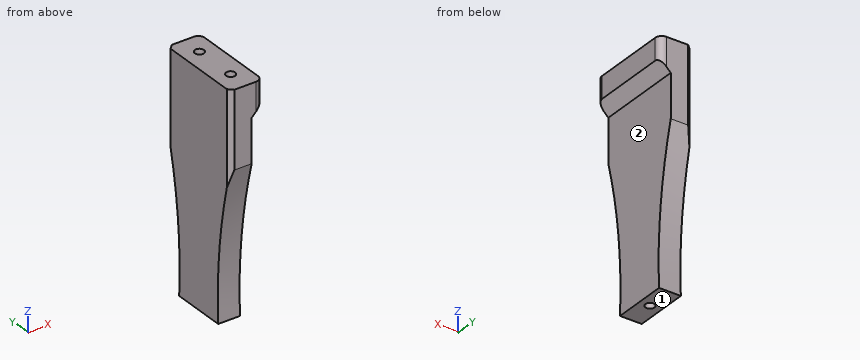
```python
from build123d import *

# Parameters (mm, degrees)
BOSS_EXTRUDE1_DEPTH   = 20
CUT_EXTRUDE1_DEPTH    = 108.935165725
FILLET2_R             = 3
M5_TAPPED_HOLE1_D     = 4.2
M5_TAPPED_HOLE1_DEPTH = 13.7381927
M5_TAPPED_HOLE1_TIP   = 1.2618073
M5_TAPPED_HOLE2_D     = 4.2
M5_TAPPED_HOLE2_DEPTH = 13.7381927
M5_TAPPED_HOLE2_TIP   = 1.2618073
CHAMFER1_SIZE         = 5
CHAMFER2_SIZE         = 2


with BuildPart() as part:
    # Sketch1 → Boss-Extrude1 (new, symmetric)
    with BuildSketch(Plane(origin=(0, 0, 0), x_dir=(1, 0, 0), z_dir=(0, 1, 0))):
        Polygon((0, 0), (15, 0), (15, 10), (10, 10), (10, 105), (0, 105), align=None)
    extrude(amount=BOSS_EXTRUDE1_DEPTH, both=True)

    # Sketch3 → Cut-Extrude1 (cut, through all)
    with BuildSketch(Plane.ZY):
        with BuildLine():
            Line((-35, -20), (-105, -20))
            Line((-105, -20), (-105, -12.5))
            add(Edge.make_bspline(
                [(-105, -12.5), (-69.476387912, -10.752287941), (-35, -20)],
                knots=[0, 0, 0, 1, 1, 1], degree=2))
        make_face()
    cut_extrude1 = extrude(amount=-CUT_EXTRUDE1_DEPTH, mode=Mode.SUBTRACT)

    # Mirror1: Cut-Extrude1 across plane
    add(cut_extrude1.mirror(Plane.ZX), mode=Mode.SUBTRACT)

    # Fillet2
    fillet2_edges = [part.edges().sort_by_distance(p)[0] for p in [
        (15, 20, -5),
        (15, -20, -5),
    ]]
    fillet(fillet2_edges, radius=FILLET2_R)

    # M5 Tapped Hole1
    with Locations(Plane(origin=(0, 0, -105), x_dir=(-1, 0, 0), z_dir=(0, 0, -1))):
        with Locations((-5.195, 0)):
            Hole(M5_TAPPED_HOLE1_D / 2, depth=M5_TAPPED_HOLE1_DEPTH)
            with Locations((0, 0, -(M5_TAPPED_HOLE1_DEPTH + M5_TAPPED_HOLE1_TIP / 2))):  # 118° drill point
                Cone(0, M5_TAPPED_HOLE1_D / 2, M5_TAPPED_HOLE1_TIP, mode=Mode.SUBTRACT)

    # M5 Tapped Hole2
    with Locations(Plane.XY):
        with Locations((7.5, -10), (7.5, 10)):
            Hole(M5_TAPPED_HOLE2_D / 2, depth=M5_TAPPED_HOLE2_DEPTH)
            with Locations((0, 0, -(M5_TAPPED_HOLE2_DEPTH + M5_TAPPED_HOLE2_TIP / 2))):  # 118° drill point
                Cone(0, M5_TAPPED_HOLE2_D / 2, M5_TAPPED_HOLE2_TIP, mode=Mode.SUBTRACT)

    # Chamfer1
    chamfer1_edges = [part.edges().sort_by_distance(p)[0] for p in [
        (10, 0, -10),
    ]]
    chamfer(chamfer1_edges, length=CHAMFER1_SIZE - 0.0001)  # a hair under: the kernel refuses the full size

    # Chamfer2
    chamfer2_edges = [part.edges().sort_by_distance(p)[0] for p in [
        (0, -20, -17.5),
        (0, 20, -17.5),
    ]]
    chamfer(chamfer2_edges, length=CHAMFER2_SIZE)


solid = part.part
```
Geometry: final body of the model. Coordinates: model frame, mm. Face numbers are marked on the shaded views. A direction names the side the tool comes from. Coordinates: 2 decimals unless noted, no trailing zeros. Loops run counter-clockwise (first coordinate to the right, second up) from the corner with the lowest first, then second, coordinate; pieces in that order, holes last. Notation, with made-up numbers: (7.25, 23.5) -> (62.25, 23.5) arc R3 ccw to (62.25, 27.5) -> close; hole circle Ø7 at (-21.75, -31). An arc over 180 degrees is marked (long way). Use a Markdown table: item, result. Add a question column.
(1) Section query B-B, the plane z = -31.5. Return loops of the section in (x, y), plus the area to 3 significant figures.
(2) Access query for the marked faces 1 and 2. Directions: +Z, -Z, +X, -X, +Y, -Y. A direction counts if a zero-diameter tool reaches every point of the face in a straight line with its end or side. Return the directions, or none.
(3) Section query C-C, the plane x = 13.75. Return loops of the section in (y, z).
(4) Line query: line 1 along Y through (x, z) = (7.5, -10.5); line 2 along X through (y, z) = (10, -3); line 3 along Z through (x, y) = (11.25, -17.5). Output: solid intervals per line, ascending.
(5) Pin query (flat end, axial travel): pin 1 Ø2 at (y, z) = (2.5, -38.5) entering from +X; pin 2 Ø8 at (x, z) = (2, -81.5) entering from +Y; pin 3 Ø1.5 at (x, z) = (6.5, -91.5) entering from -Y. Return the tip coordinate at first contact, or that it passes through.
Answer:
| question | item | result |
|---|---|---|
| 1 | outline | (0, -18) -> (2, -20) -> (10, -20) -> (10, 20) -> (2, 20) -> (0, 18) -> close |
| 1 | area | 396 mm^2 |
| 2 | face 1 | -Z, +X, -X, +Y, -Y |
| 2 | face 2 | -Z, +X, +Y, -Y |
| 3 | outline | (-19.44, -11.25) -> (19.44, -11.25) -> (19.44, 0) -> (-19.44, 0) -> close |
| 4 | line 1 | y = -20 to -12.1, -7.9 to 7.9, 12.1 to 20 |
| 4 | line 2 | x = 0 to 5.4, 9.6 to 15 |
| 4 | line 3 | z = -13.75 to 0 |
| 5 | pin 1 | stops at x = 10 |
| 5 | pin 2 | stops at y = 12.81 |
| 5 | pin 3 | stops at y = -12.24 |
